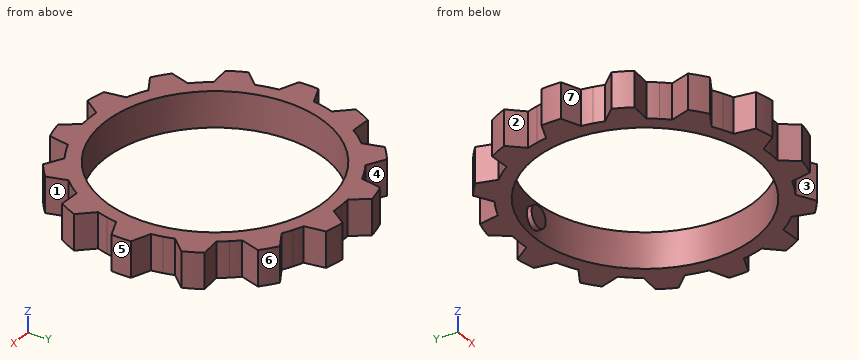
from build123d import *

# Parameters (mm, degrees)
SKETCH1_R           = 20
SKETCH1_R_2         = 15.5
BOSS_EXTRUDE1_DEPTH = 2.5
CUT_EXTRUDE1_DEPTH  = 5
CIRPATTERN1_COUNT   = 14
SKETCH6_R           = 1.5
BOSS_EXTRUDE2_DEPTH = 0.75


with BuildPart() as part:
    # Sketch1 → Boss-Extrude1 (new, symmetric)
    with BuildSketch(Plane.XY):
        Circle(SKETCH1_R)
        Circle(SKETCH1_R_2, mode=Mode.SUBTRACT)
    extrude(amount=BOSS_EXTRUDE1_DEPTH, both=True)

    # Sketch2 → Cut-Extrude1 (cut)
    with BuildSketch(Plane.XY.offset(2.5)):
        with BuildLine():
            ThreePointArc((-1.5, 17.435595774), (-0.750690999, 17.48389153), (0, 17.5))
            Line((0, 17.5), (0, 20))
            ThreePointArc((0, 20), (-1.566688393, 19.938542762), (-3.123748353, 19.754548748))
            Line((-3.123748353, 19.754548748), (-1.5, 17.435595774))
        make_face()
        with BuildLine():
            Line((0, 20), (0, 17.5))
            ThreePointArc((0, 17.5), (0.750690999, 17.48389153), (1.5, 17.435595774))
            Line((1.5, 17.435595774), (3.123748353, 19.754548748))
            ThreePointArc((3.123748353, 19.754548748), (1.566688393, 19.938542762), (0, 20))
        make_face()
    cut_extrude1 = extrude(amount=-CUT_EXTRUDE1_DEPTH, mode=Mode.SUBTRACT)

    # CirPattern1: Cut-Extrude1 ×14 about axis
    cirpattern1_axis = Axis((0, 0, 0), (0, 0, 1))
    for i in range(1, CIRPATTERN1_COUNT):
        add(cut_extrude1.rotate(cirpattern1_axis, i * 360 / CIRPATTERN1_COUNT), mode=Mode.SUBTRACT)

    # Sketch6 → Boss-Extrude2 (add)
    with BuildSketch(Plane(origin=(0, 15.5, 0), x_dir=(1, 0, 0), z_dir=(0, 1, 0))):
        with Locations(Location((0, 0, 0), (0, 0, 270))):
            Circle(SKETCH6_R)
    extrude(amount=-BOSS_EXTRUDE2_DEPTH)


solid = part.part
Could you check a few things on this model? Use its own coordinates, in mm. Face numbers are marked on the shaded views. A direction names the side the tool comes from. Coordinates: 2 decimals unless noted, no trailing zeros. Order: outer loops, then holes, each group sorted by start corner. A loop starts at its lowest first (then second) coordinate and runs counter-clockwise, first axis right, second up. Notation, with made-up numbers: (54.5, 13) - (104.5, 13) arc R37 ccw to (104.5, 51) - close; hole circle Ø3 at (81, -25.5). An arc over 180 degrees is marked (long way). Answer in a Markdown table with one row per item. Add a question column.
(1) On a 3-axis mill with a long thin cutter (end or side, diameter ignored), from which of +Z, -Z, +X, -X, +Y, -Y can I reach the whole of each face in a straight line? I mean the marked faces 1, 2, 3 and 4. Say none if no direction works.
(2) If we section it at B-B, the plane x = 10: Please give me the cut outline in (y, z).
(3) I need wall thicknesses on L1, parallel to Y at x = -17.5, z = -0.5; L2, parallel to Y at x = 18, z = -0.15; L3, parallel to X at y = -14, z = 0.45. Which ranges of each line are inside material? Lowest first, please.
(4) Will these pins go through, and if not, where does the flat tip stop? pin 1 (1.5 mm diameter, centred on x = -12, z = -1, fed in from +Y); pin 2 (0.9 mm diameter, centred on x = -0.5, z = 0, fed in from -Y); pin 3 (2 mm diameter, centred on x = -5.5, z = 0.5, fed in from -Y); pin 4 (4 mm diameter, centred on x = 11.5, y = 3, fed in from +Z).
(5) If we section it at A-A, the plane y = 0: Please give me the cut outline in (x, z).
(6) If we mould it in two halves opening along Y, with no side actions, what happens to the marked faces 5, 6 and 7? For each: released by +Y, released by -Y, zero draft, split by the parting line, or undercut.
Results are:
| question | item | result |
|---|---|---|
| 1 | face 1 | +Z, -Z, +X |
| 1 | face 2 | +Z, -Z, -X |
| 1 | face 3 | +Z, -Z, -Y |
| 1 | face 4 | +Z, -Z, +Y |
| 2 | outline | (-15.67, -2.5) - (-11.84, -2.5) - (-11.84, 2.5) - (-15.67, 2.5) - close; (11.84, -2.5) - (15.67, -2.5) - (15.67, 2.5) - (11.84, 2.5) - close |
| 3 | L1 | y = -9.68 to -6.27, -2.35 to 2.35, 6.27 to 9.68 |
| 3 | L2 | y = -8.72 to -6.82, -2.15 to 2.15, 6.82 to 8.72 |
| 3 | L3 | x = -13.27 to -6.65, 6.65 to 13.27 |
| 4 | pin 1 | stops at y = 16.44 |
| 4 | pin 2 | stops at y = -17.5 |
| 4 | pin 3 | stops at y = -19.49 |
| 4 | pin 4 | passes through |
| 5 | outline | (-20, -2.5) - (-15.5, -2.5) - (-15.5, 2.5) - (-20, 2.5) - close; (15.5, -2.5) - (20, -2.5) - (20, 2.5) - (15.5, 2.5) - close |
| 6 | face 5 | split by the parting line |
| 6 | face 6 | released by +Y |
| 6 | face 7 | undercut |
